Autodesk Inventor part; units mm, degrees
ref_plane "YZ Plane" through (0, 0, 0) normal (1, 0, 0) x (0, 1, 0)
ref_plane "XZ Plane" through (0, 0, 0) normal (0, 1, 0) x (-1, 0, 0)
ref_plane "XY Plane" through (0, 0, 0) normal (0, 0, 1) x (1, 0, 0)
sketch "Esboço1" plane through (0, 0, 0) normal (0, 1, 0) x (-1, 0, 0)
  line L0 (0, 100) -> (50, 100)
  line L1 (50, 100) -> (75.8622, 84.7964)
  line L2 (50, 100) -> (80, 100) construction
  line L3 (75.8622, 84.7964) -> (75.8622, 67.7964)
  line L4 (75.8622, 67.7964) -> (117.8622, 67.7964)
  line L5 (117.8622, 67.7964) -> (170.8622, 67.7964) construction
  circle A0 centre (68.629, 76.2964) radius 2.5
  circle A1 centre (58.629, 76.2964) radius 2.5
  circle A2 centre (48.629, 76.2964) radius 2.5
  circle A3 centre (38.629, 76.2964) radius 2.5
  line L6 (0, -100) -> (50, -100)
  line L7 (50, -100) -> (75.8622, -84.7964)
  line L8 (75.8622, -84.7964) -> (75.8622, -67.7964)
  line L9 (75.8622, -67.7964) -> (117.8622, -67.7964)
  circle A4 centre (68.629, -76.2964) radius 2.5
  circle A5 centre (58.629, -76.2964) radius 2.5
  circle A6 centre (48.629, -76.2964) radius 2.5
  circle A7 centre (38.629, -76.2964) radius 2.5
  line L10 (0, 100) -> (0, -100)
  line L11 (75.8622, -82.1665) -> (75.8622, -70.1665)
  circle A8 centre (61.129, 0) radius 23
  line L12 (117.8622, 67.7964) -> (139.8134, 26.55)
  line L13 (117.8622, -67.7964) -> (139.8134, -26.55)
  line L14 (139.8134, 26.55) -> (139.8134, -26.55)
  line L15 (0, 0) -> (61.129, 0)
  circle A9 centre (59.9305, 27.5032) radius 1.5
  circle A10 centre (60.6516, -27.5032) radius 1.5
  dimension "d5" = 30
  dimension "d6" = 30.45
  dimension "d17" = 10
  dimension "d32" = 42
  dimension "d33" = 25.8621
  dimension "d34" = 50
  dimension "d37" = 46
  dimension "d40" = 53.1001
  dimension "d41" = 21.9513
  dimension "d42" = 17
  dimension "d43" = 46.7239
  dimension "d44" = 118.022
  dimension "d45" = 61.129
  dimension "d46" = 200
  dimension "d48" = 3
  dimension "d53" = 3
extrude "Extrusão1" add sketch "Esboço1" along normal blind 1 contours A8 | L0 L1 L3 L4 L12 L14 L13 L9 L8 L7 L6 L10 | A9 | A10
sketch "Esboço3" plane through (0, 1, 0) normal (0, 1, 0) x (1, 0, 0)
  circle A0 centre (-60.4361, 0) radius 23.1709
  point P0 (0, 0)
extrude "Extrusão3" cut sketch "Esboço3" against normal blind 3.75
extrude "Extrusão4" cut sketch "Esboço1" along normal blind 3.75 contours A9
extrude "Extrusão5" [suppressed]
extrude "Extrusão6" cut sketch "Esboço1" along normal blind 3.75 contours A10
sketch "Esboço4" plane through (0, 1, 0) normal (0, 1, 0) x (1, 0, 0)
  point P0 (0, 0)
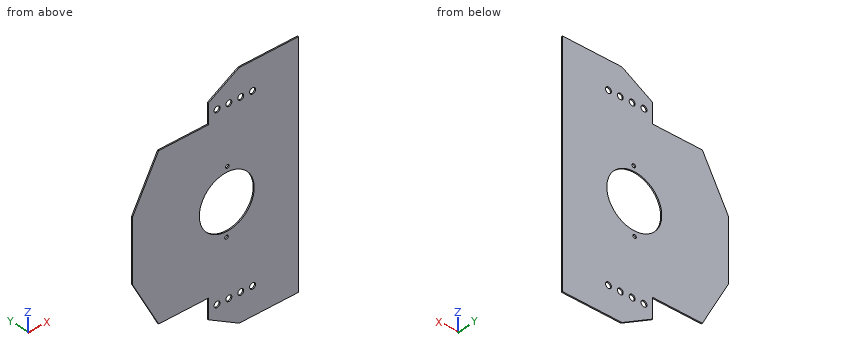
The listing builds one solid part. Answer for the finished solid, in the listing's coordinates (mm). Round coordinates to 2 decimals unless told otherwise and drop trailing zeros. Order: outer loops, then holes, each group sorted by start corner. A loop starts at its lowest first (then second) coordinate and runs counter-clockwise, first axis right, second up. Notation, with made-up numbers: (33, 60) -> (82, 60) arc R20 cw to (82, 68) -> close; hole circle Ø8 at (88.25, -37.5). An arc over 180 degrees is marked (long way). Answer as CSV lines item,"result".
Q1. Consider line 1 (X direction, y = 0.8, z = 76.5); line 2 (Z direction, x = -73, y = 0.25); line 3 (Z direction, x = -42.5, y = 0.4). Determine where each line is inside the solid, lowest interval first. Write a range as from..to.
Computed values:
line 1,"x = -75.86..-71.12, -66.14..-61.12, -56.14..-51.12, -46.14..-41.12, -36.14..0"
line 2,"z = -86.48..-19.47, 19.47..86.48"
line 3,"z = -100..-14.67, 14.67..100"
Q2. A cutting plane is placed at A-A on z = 0. Determine the outline of the cut face in (x, y).
Computed values:
outline,"(-139.81, 0) -> (-83.61, 0) -> (-83.61, 1) -> (-139.81, 1) -> close; (-37.27, 0) -> (0, 0) -> (0, 1) -> (-37.27, 1) -> close"
Q3. Given pin 1 (0.5 mm diameter, centred on x = -89.5, y = 0.5, fed in from -Z), flat-ended and moving along its own axis, determine where the tip first touches the part or whether it passes through.
Computed values:
pin 1,"stops at z = -67.8"
Q4. A cutting plane is placed at D-D on x = -123.5. Determine the outline of the cut face in (y, z), plus the area to 3 significant figures.
Computed values:
outline,"(0, -57.2) -> (1, -57.2) -> (1, 57.2) -> (0, 57.2) -> close"
area,"114 mm^2"
Q5. A cutting plane is placed at C-C on x = -80.5. Determine the outline of the cut face in (y, z), plus the area to 3 significant figures.
Computed values:
outline,"(0, -67.8) -> (1, -67.8) -> (1, -11.59) -> (0, -11.59) -> close; (0, 11.59) -> (1, 11.59) -> (1, 67.8) -> (0, 67.8) -> close"
area,"112 mm^2"
Q6. A cutting plane is placed at B-B on y = 0.2. Give the number of separate pieces and of enclosed holes in the cut face, plus the area to 3 significant figures.
Computed values:
separate pieces,"1"
enclosed holes,"11"
area,"20,700 mm^2"
